```python
from build123d import *

# Parameters (mm, degrees)
SKETCH_1_R          = 12.5
SKETCH_1_R_2        = 2.5
EXTRUDE_1_DEPTH     = 8
SKETCH_2_R          = 7.5
SKETCH_2_R_2        = 2.5
EXTRUDE_2_DEPTH     = 8
SKETCH_4_R          = 1.5
CUT_EXTRUDE_1_DEPTH = 10


with BuildPart() as part:
    # Эскиз1 → Бобышка-Вытянуть1 (new body)
    with BuildSketch(Plane.XY):
        Circle(SKETCH_1_R)
        Circle(SKETCH_1_R_2, mode=Mode.SUBTRACT)
    extrude(amount=EXTRUDE_1_DEPTH)

    # Эскиз2 → Бобышка-Вытянуть2 (add)
    with BuildSketch(Plane.XY.offset(8)):
        Circle(SKETCH_2_R)
        Circle(SKETCH_2_R_2, mode=Mode.SUBTRACT)
    extrude(amount=EXTRUDE_2_DEPTH)

    # Эскиз4 → Вырез-Вытянуть1 (cut)
    with BuildSketch(Plane(origin=(0, 0, 0), x_dir=(0, 0, -1), z_dir=(1, 0, 0))):
        with Locations((-11, 0)):
            Circle(SKETCH_4_R)
    extrude(amount=-CUT_EXTRUDE_1_DEPTH, mode=Mode.SUBTRACT)


solid = part.part
```
Check sheet for the modelled part. Datum: model origin and axes. Units: mm. A direction names the side the tool comes from. Coordinates: 2 decimals unless noted, no trailing zeros. Write each loop counter-clockwise with the first axis right and the second up, starting at its lowest first coordinate (ties: lowest second). Pieces come first, ordered by that corner, then holes. Notation, with made-up numbers: (28, -34.75) -> (84, -34.75) arc R19 cw to (84, -8.75) -> close; hole circle Ø9 at (66.25, 5). An arc over 180 degrees is marked (long way). Use a Markdown table: item, result.
1. Tool access check on faces 1 (the cylindrical face through (2.385, 0.751, 7.888)), 2 (the cylindrical face through (6.93, -2.87, 11.94)). Record the directions out of +Z, -Z, +X, -X, +Y, -Y that give a thin tool (end or side, any length) a straight path to the whole face; none if there is none.
Reported:
| item | result |
|---|---|
| face 1 | +Z, -Z |
| face 2 | +Z |
2. Sectioned sample at B-B (x = 0). Enter the section's corners in (y, z).
Reported:
| item | result |
|---|---|
| outline | (-12.5, 0) -> (-2.5, 0) -> (-2.5, 16) -> (-7.5, 16) -> (-7.5, 8) -> (-12.5, 8) -> close; (2.5, 0) -> (12.5, 0) -> (12.5, 8) -> (7.5, 8) -> (7.5, 16) -> (2.5, 16) -> close |
3. Release check for a two-part mould opening along Z. For faces 3 (the flat face through (0, -3, 0)), 4 (the flat face through (0, -8, 8)), 5 (the cylindrical face through (11.923, 3.755, 3.944)), 6 (the cylindrical face through (-4.712, -0.575, 9.614)) record: pulls with the +Z half, pulls with the -Z half, needs draft (parallel to the pull), parting line crosses it, or undercut.
Reported:
| item | result |
|---|---|
| face 3 | pulls with the -Z half |
| face 4 | pulls with the +Z half |
| face 5 | needs draft |
| face 6 | undercut |
4. Scan lines: line 1 along X through (y, z) = (0, 8.5); line 2 along Z through (x, y) = (7, -4.5). Record each from-to range of solid material in increasing order.
Reported:
| item | result |
|---|---|
| line 1 | x = -7.5 to -2.5, 2.5 to 7.5 |
| line 2 | z = 0 to 8 |
5. Go/stop test with flat-tipped pins: pin 1 Ø3 at (x, z) = (6, 2) entering from +Y; pin 2 Ø2 at (x, z) = (-3.5, 11.5) entering from -Y; pin 3 Ø1.5 at (x, z) = (1.5, 13.5) entering from +Y. Record where each tip stops, or that it passes through.
Reported:
| item | result |
|---|---|
| pin 1 | stops at y = 11.66 |
| pin 2 | stops at y = -7.07 |
| pin 3 | stops at y = 7.46 |
6. Sectioned sample at D-D (x = -5.5). Enter the section's corners in (y, z).
Reported:
| item | result |
|---|---|
| outline | (-11.22, 0) -> (11.22, 0) -> (11.22, 8) -> (5.1, 8) -> (5.1, 16) -> (-5.1, 16) -> (-5.1, 8) -> (-11.22, 8) -> close; hole circle Ø3 at (0, 11) |
7. Sectioned sample at A-A (y = 0). Enter the section's corners in (x, z).
Reported:
| item | result |
|---|---|
| outline | (-12.5, 0) -> (-2.5, 0) -> (-2.5, 9.5) -> (-7.5, 9.5) -> (-7.5, 8) -> (-12.5, 8) -> close; (-7.5, 12.5) -> (-2.5, 12.5) -> (-2.5, 16) -> (-7.5, 16) -> close; (2.5, 0) -> (12.5, 0) -> (12.5, 8) -> (7.5, 8) -> (7.5, 16) -> (2.5, 16) -> close |
8. Sectioned sample at C-C (z = 6). Enter the section's corners in (x, y).
Reported:
| item | result |
|---|---|
| outline | circle Ø25 at (0, 0); hole circle Ø5 at (0, 0) |
